```python
from build123d import *

# Parameters (mm, degrees)
F0_W     = 229.6963825016
F0_H     = 108.4231149972
F0_R     = 9.942969978
F0_R_2   = 8.7794022154
F1_DEPTH = 152.4
F2_R     = 15.637009349
F2_R_2   = 15.3013139209
F3_DEPTH = 108.4241150972
F4_R     = 12.7


with BuildPart() as f1:
    # F0 (on Right) → F1 (new body, symmetric)
    with BuildSketch(Plane.YZ):
        Rectangle(F0_W, F0_H)
        with BuildLine():
            ThreePointArc((-43.4804819524, -25.5854520947), (-61.6064477727, -33.2849477454), (-57.3824048042, -14.049815014))
            add(Edge.make_bspline(
                [(-57.3824048042, -14.049815014), (-42.3782414018, -9.9389745723), (-14.222776702, -2.224940818), (-34.1653761162, -18.1479024622), (-43.4804819524, -25.5854520947)],
                knots=[0, 0, 0, 0, 0.5329041294, 1, 1, 1, 1], degree=3))
        make_face(mode=Mode.SUBTRACT)
        with Locations((-63.2981136441, 26.1770226061)):
            Circle(F0_R, mode=Mode.SUBTRACT)
        with Locations((28.9869904518, 24.9938834459)):
            Circle(F0_R_2, mode=Mode.SUBTRACT)
    extrude(amount=F1_DEPTH, both=True)

    # F2 (on face) → F3 (cut, through all)
    with BuildSketch(Plane.XY.offset(54.2115574986)):
        with Locations((-114.2957806332, 79.1441154076)):
            Circle(F2_R)
        with Locations((63.5042193668, 62.5812566792)):
            Circle(F2_R_2)
        with BuildLine():
            ThreePointArc((-0.654293087, -21.5848963512), (33.3430248824, -50.0341097243), (63.7498454838, -17.775767678))
            ThreePointArc((63.7498454838, -17.775767678), (48.9743135647, 9.3649362096), (18.1596027821, 11.6860890263))
            ThreePointArc((18.1596027821, 11.6860890263), (20.7182170411, 6.0902653943), (21.5948107177, 0))
            ThreePointArc((21.5948107177, 0), (15.0367302723, -15.4994384625), (-0.654293087, -21.5848963512))
        make_face()
        with BuildLine():
            ThreePointArc((21.5948107177, 0), (20.7182170411, 6.0902653943), (18.1596027821, 11.6860890263))
            ThreePointArc((18.1596027821, 11.6860890263), (3.3062432367, -1.8695964447), (-0.654293087, -21.5848963512))
            ThreePointArc((-0.654293087, -21.5848963512), (15.0367302723, -15.4994384625), (21.5948107177, 0))
        make_face()
        with BuildLine():
            ThreePointArc((-0.654293087, -21.5848963512), (3.3062432367, -1.8695964447), (18.1596027821, 11.6860890263))
            ThreePointArc((18.1596027821, 11.6860890263), (-18.7975685629, 10.6295468416), (-0.654293087, -21.5848963512))
        make_face()
    extrude(amount=-F3_DEPTH, mode=Mode.SUBTRACT)

    # F4
    f4_edges = [f1.edges().sort_by_distance(p)[0] for p in [
        (0, 114.848191, 54.211557),
    ]]
    fillet(f4_edges, radius=F4_R)


solid = f1.part
```
Design review of the part built by this model. Coordinates are the model's own, in mm. Coordinates: 2 decimals unless noted, no trailing zeros. Order: outer loops, then holes, each group sorted by start corner. A loop starts at its lowest first (then second) coordinate and runs counter-clockwise, first axis right, second up.
1) Take a section at B-B, the plane y = 68. Give the boundary of the cut face in (x, z), and give its area (3 significant figures).
2) Take a section at D-D, the plane x = 94.5. State how many separate pieces and enclosed holes the cut face has, and give its area (3 significant figures).
3) Take a section at C-C, the plane z = -46. Give the boundary of the cut face in (x, y).
4) Mouldability with a two-part tool opening along Z and no side actions: class faces 1 (the flat face through (152.4, -2, 1)), 2 (the cylindrical face through (-2.13, -71.19, 20.13)), 3 (the flat face through (2, 24, -54.212)) as +Z half, -Z half, draft (parallel to the pull), parting line (faces both ways), or undercut.
5) Clearance check with a flat-ended pin moving along its axis: pin 1 (12 mm diameter, centred on y = -63.3, z = 26.18, fed in from +X). State where the tip first meets the part, or that it passes through.
6) Wall thickness on line 1 along Y through (x, z) = (105, 25.5); line 2 along Y through (x, z) = (56.5, 33); line 3 along X through (y, z) = (66.5, -35): over which ranges is each line inside the solid? List them lowest first.
7) Take a section at A-A, the plane y = 0. Give the boundary of the cut face in (x, z), and give its area (3 significant figures).
Returned:
1. outline: (-152.4, -54.21) - (-125.27, -54.21) - (-125.27, 54.21) - (-152.4, 54.21) - close; (-103.33, -54.21) - (49.19, -54.21) - (49.19, 54.21) - (-103.33, 54.21) - close; (77.81, -54.21) - (152.4, -54.21) - (152.4, 54.21) - (77.81, 54.21) - close
1. area: 27,600 mm2
2. separate pieces: 1
2. enclosed holes: 3
2. area: 23,700 mm2
3. outline: (-152.4, -114.85) - (152.4, -114.85) - (152.4, 114.85) - (-152.4, 114.85) - close; hole circle Ø31.27 at (-114.3, 79.14); hole (-0.65, -21.58) arc R32.31 ccw (long way) to (18.16, 11.69) arc R21.59 ccw (long way) to start; hole circle Ø30.6 at (63.5, 62.58)
4. face 1: draft
4. face 2: undercut
4. face 3: -Z half
5. pin 1: passes through
6. line 1: y = -114.85 to -73.22, -53.38 to 20.22, 37.75 to 114.85
6. line 2: y = -114.85 to -70.53, -56.07 to -38.17, 2.62 to 25.38, 32.59 to 48.98, 76.19 to 114.85
6. line 3: x = -152.4 to -123.5, -105.1 to 48.71, 78.3 to 152.4
7. outline: (-152.4, -54.21) - (-21.59, -54.21) - (-21.59, 54.21) - (-152.4, 54.21) - close; (58.42, -54.21) - (152.4, -54.21) - (152.4, 54.21) - (58.42, 54.21) - close
7. area: 24,400 mm2
